Design review of the part built by this model. Coordinates are the model's own, in mm. A direction names the side the tool comes from. Coordinates: 2 decimals unless noted, no trailing zeros. Write each loop counter-clockwise with the first axis right and the second up, starting at its lowest first coordinate (ties: lowest second). Pieces come first, ordered by that corner, then holes.
```python
from build123d import *

# Parameters (mm, degrees)
ESQUISSE1_W                  = 156
ESQUISSE1_H                  = 84
BOSS_EXTRU_1_DEPTH           = 59
ESQUISSE2_W                  = 78
ESQUISSE2_H                  = 16
ESQUISSE2_W_2                = 7
ESQUISSE2_H_2                = 35
ESQUISSE2_W_3                = 4.2
ESQUISSE2_H_3                = 2.5
ENL_V_MAT_EXTRU_1_DEPTH      = 177.572550515
ENL_V_MAT_EXTRU_3_DEPTH      = 141.546285889
ESQUISSE4_W                  = 52
ESQUISSE4_H                  = 20
ENL_V_MAT_EXTRU_4_DEPTH      = 59
BOSS_EXTRU_2_DEPTH           = 34
ESQUISSE6_W                  = 95
ESQUISSE6_H                  = 3
BOSS_EXTRU_3_DEPTH           = 34
ESQUISSE8_R                  = 2.1
ENL_V_MAT_EXTRU_5_DEPTH      = 37
BOSS_EXTRU_4_DEPTH           = 3
ENL_V_MAT_EXTRU_6_DEPTH      = 30
ENL_V_MAT_EXTRU_6_DEPTH_BACK = 10
ESQUISSE10_W                 = 9.584266769
ESQUISSE10_H                 = 152
ESQUISSE11_W                 = 85.415733231
ESQUISSE11_H                 = 1
ENL_V_MAT_EXTRU_7_DEPTH      = 10


with BuildPart() as part:
    # Esquisse1 → Boss.-Extru.1 (new body)
    with BuildSketch(Plane(origin=(0, 0, 0), x_dir=(1, 0, 0), z_dir=(0, 1, 0))):
        with Locations((23.701811573, 15.972972973)):
            Rectangle(ESQUISSE1_W, ESQUISSE1_H)
    extrude(amount=BOSS_EXTRU_1_DEPTH)

    # Esquisse2 → Enlèv. mat.-Extru.1 (cut, through all)
    with BuildSketch(Plane(origin=(101.701811573, 0, 0), x_dir=(0, 0, -1), z_dir=(1, 0, 0))):
        Polygon((15.972972973, 24), (47.972972973, 24), (47.972972973, 56), (-16.027027027, 56), (-16.027027027, 24), align=None)
        with Locations((15.972972973, 13)):
            Rectangle(ESQUISSE2_W, ESQUISSE2_H)
        with Locations((-22.527027027, 41.5)):
            Rectangle(ESQUISSE2_W_2, ESQUISSE2_H_2)
        Polygon((54.972972973, 24), (57.972972973, 24), (57.972972973, 59), (50.972972973, 59), (50.972972973, 24), align=None)
        with Locations((24.072972973, 1.25)):
            Rectangle(ESQUISSE2_W_3, ESQUISSE2_H_3)
    extrude(amount=-ENL_V_MAT_EXTRU_1_DEPTH, mode=Mode.SUBTRACT)

    # Esquisse3 → Enlèv. mat.-Extru.3 (cut, through all)
    with BuildSketch(Plane.XY.offset(19.027027027)):
        with BuildLine():
            Line((101.701811573, 59), (40.701811573, 59))
            add(Edge.make_bspline(
                [(40.701811573, 59), (63.23269898, 27.796698054), (101.701811573, 24)],
                knots=[0, 0, 0, 1, 1, 1], degree=2))
            Line((101.701811573, 24), (101.701811573, 59))
        make_face()
    extrude(amount=-ENL_V_MAT_EXTRU_3_DEPTH, mode=Mode.SUBTRACT)

    # Esquisse4 → Enlèv. mat.-Extru.4 (cut)
    with BuildSketch(Plane.XY.offset(19.027027027)):
        with Locations((-25.298188427, 34)):
            Rectangle(ESQUISSE4_W, ESQUISSE4_H)
    extrude(amount=-ENL_V_MAT_EXTRU_4_DEPTH, mode=Mode.SUBTRACT)

    # Esquisse5 → Boss.-Extru.2 (add)
    with BuildSketch(Plane(origin=(0, 0, -57.972972973), x_dir=(-1, 0, 0), z_dir=(0, 0, -1))):
        Polygon((-101.701811573, 2.5), (-40.701811573, 2.75), (-40.701811573, 5.5), (-101.701811573, 5.5), align=None)
        Polygon((-40.701811573, 2.75), (-6.701811573, 2.660526316), (-6.701811573, 5.5), (-40.701811573, 5.5), align=None)
    extrude(amount=BOSS_EXTRU_2_DEPTH)

    # Esquisse6 → Boss.-Extru.3 (add)
    with BuildSketch(Plane.XY.offset(26.027027027)):
        with Locations((54.201811573, 4)):
            Rectangle(ESQUISSE6_W, ESQUISSE6_H)
    extrude(amount=BOSS_EXTRU_3_DEPTH)

    # Esquisse8 → Enlèv. mat.-Extru.5 (cut)
    with BuildSketch(Plane(origin=(0, 5.5, 0), x_dir=(1, 0, 0), z_dir=(0, 1, 0))):
        with Locations(Location((16.701811573, -50.027027027, 0), (0, 0, 180))):
            Circle(ESQUISSE8_R)
        with Locations(Location((91.701811573, -50.027027027, 0), (0, 0, 180))):
            Circle(ESQUISSE8_R)
        with Locations(Location((16.701811573, 81.972972973, 0), (0, 0, 180))):
            Circle(ESQUISSE8_R)
        with Locations(Location((91.701811573, 81.972972973, 0), (0, 0, 180))):
            Circle(ESQUISSE8_R)
    extrude(amount=-ENL_V_MAT_EXTRU_5_DEPTH, mode=Mode.SUBTRACT)

    # Esquisse9 → Boss.-Extru.4 (add)
    with BuildSketch(Plane.ZY.offset(54.298188427)):
        Polygon((-57.972972973, 0), (-57.972972973, 24), (-50.972972973, 24), (-50.972972973, 59), (19.027027027, 59), (19.027027027, 24), (26.027027027, 24), (26.027027027, 0), (-21.972972973, 0), (-21.972972973, 2.5), (-26.172972973, 2.5), (-26.172972973, 0), align=None)
    extrude(amount=BOSS_EXTRU_4_DEPTH)

    # Esquisse10 → Enlèv. mat.-Extru.6 (cut, two sides: drawn at the far end of the back side and taken through both)
    with BuildSketch(Plane(origin=(0, 5.5, 0), x_dir=(1, 0, 0), z_dir=(0, 1, 0)).offset(-ENL_V_MAT_EXTRU_6_DEPTH_BACK)):
        with Locations((96.909678189, 15.972972973)):
            Rectangle(ESQUISSE10_W, ESQUISSE10_H)
    extrude(amount=ENL_V_MAT_EXTRU_6_DEPTH + ENL_V_MAT_EXTRU_6_DEPTH_BACK, mode=Mode.SUBTRACT)

    # Esquisse11 → Enlèv. mat.-Extru.7 (cut)
    with BuildSketch(Plane(origin=(0, 5.5, 0), x_dir=(1, 0, 0), z_dir=(0, 1, 0))):
        with Locations((49.409678189, 91.472972973)):
            Rectangle(ESQUISSE11_W, ESQUISSE11_H)
        with Locations((49.409678189, -59.527027027)):
            Rectangle(ESQUISSE11_W, ESQUISSE11_H)
    extrude(amount=-ENL_V_MAT_EXTRU_7_DEPTH, mode=Mode.SUBTRACT)


solid = part.part
```
(1) Consider section A-A (x = -10.5). Give the boundary of the cut face in (y, z).
(2) Mouldability with a two-part tool opening along Z and no side actions: class faces 5 (the flat face through (18, 12, 26.027)), 6 (the flat face through (4, 40, -47.973)), 7 (the flat face through (-5, 56, -16)), 8 (the flat face through (49, 5.5, -74)) as +Z half, -Z half, draft (parallel to the pull), parting line (faces both ways), or undercut.
(3) Wall thickness on line 1 (Y direction, x = 25, z = -38); line 2 (Y direction, x = 32, z = -24.5); line 3 (Z direction, x = -11.5, y = 13.5): over which ranges is each line inside the solid? List them lowest first.
(4) For faces 1 (the flat face through (2, 41, -50.973)), 2 (the flat face through (18, 2.5, -24)), 3 (the flat face through (-54.298, 40, -16)), 4 (the flat face through (18, 42, 19.027)), list the 3-axis set-ups (+Z, -Z, +X, -X, +Y, -Y) from which the entire face can be reached by the end or side of a thin tool; tool diameter is ignored.
(5) Insertion check: pin 1 Ø3 at (y, z) = (3.5, -74.5) entering from -X; pin 2 Ø1.2 at (x, y) = (5, 2) entering from +Z; pin 3 Ø16.5 at (x, z) = (40.5, 35.5) entering from +Y; pin 4 Ø1 at (y, z) = (7.5, -61.5) entering from -X. Each pin has a flat end and moves straight along its axis. Give the tip position at first contact, or say it passes through.
(6) Consider section D-D (x = 27). Give the boundary of the cut face in (y, z).
(7) Consider section B-B (y = 18). Give the boundary of the cut face in (x, z).
(8) Consider section C-C (z = -74.5). Give the boundary of the cut face in (x, y).
Results:
1. outline: (0, -57.97) - (24, -57.97) - (24, -50.97) - (59, -50.97) - (59, 19.03) - (44, 19.03) - (44, 16.03) - (56, 16.03) - (56, -47.97) - (24, -47.97) - (24, 26.03) - (0, 26.03) - (0, -21.97) - (2.5, -21.97) - (2.5, -26.17) - (0, -26.17) - close; hole (5, -54.97) - (21, -54.97) - (21, 23.03) - (5, 23.03) - close
2. face 5: +Z half
2. face 6: undercut
2. face 7: undercut
2. face 8: draft
3. line 1: y = 0 to 5, 21 to 24, 56 to 59
3. line 2: y = 2.5 to 5, 21 to 24, 56 to 59
3. line 3: z = -57.97 to -54.97, 23.03 to 26.03
4. face 1: -Z, +X, -X, +Y
4. face 2: +X, -X, -Y
4. face 3: +X
4. face 4: +Z, +X, -X, +Y
5. pin 1: stops at x = 6.7
5. pin 2: stops at z = 26.03
5. pin 3: stops at y = 5.5
5. pin 4: passes through
6. outline: (0, -57.97) - (2.71, -57.97) - (2.71, -90.97) - (5.5, -90.97) - (5.5, -57.97) - (24, -57.97) - (24, -50.97) - (59, -50.97) - (59, 19.03) - (24, 19.03) - (24, 26.03) - (5.5, 26.03) - (5.5, 59.03) - (2.5, 59.03) - (2.5, 26.03) - (0, 26.03) - (0, -21.97) - (2.5, -21.97) - (2.5, -26.17) - (0, -26.17) - close; hole (5, -54.97) - (21, -54.97) - (21, 23.03) - (5, 23.03) - close; hole (24, -47.97) - (56, -47.97) - (56, 16.03) - (24, 16.03) - close
7. outline: (-57.3, -57.97) - (92.12, -57.97) - (92.12, -54.97) - (-54.3, -54.97) - (-54.3, 23.03) - (92.12, 23.03) - (92.12, 26.03) - (-57.3, 26.03) - close
8. outline: (6.7, 2.66) - (40.7, 2.75) - (92.12, 2.54) - (92.12, 5.5) - (6.7, 5.5) - close
